```python
from build123d import *

# Parameters (mm, degrees)
BOSS_EXTRUDE1_DEPTH      = 1.5
BOSS_EXTRUDE2_DEPTH      = 18
BOSS_EXTRUDE2_DEPTH_BACK = 1
CUT_EXTRUDE2_DEPTH       = 2
CUT_EXTRUDE3_DEPTH       = 47.778734485
CHAMFER1_SIZE            = 1
CHAMFER2_SIZE            = 2


with BuildPart() as part:
    # Sketch1 → Boss-Extrude1 (new body)
    with BuildSketch(Plane(origin=(0, 0, 0), x_dir=(1, 0, 0), z_dir=(0, 1, 0))):
        Polygon((0, -2.84), (0, 0), (37, 0), (37, -6), (29, -6), (29, -10), (37, -10), (37, -16), (29, -16), (29, -28), (3, -28), (3, -2.84), align=None)
    extrude(amount=BOSS_EXTRUDE1_DEPTH)

    # Sketch2 → Boss-Extrude2 (add, two sides: drawn at the far end of the back side and taken through both)
    with BuildSketch(Plane(origin=(0, 1.5, 0), x_dir=(1, 0, 0), z_dir=(0, 1, 0)).offset(-BOSS_EXTRUDE2_DEPTH_BACK)):
        Polygon((7, 0), (0, 0), (0, -2.84), (3, -2.84), (3, -28), (7, -28), align=None)
    extrude(amount=BOSS_EXTRUDE2_DEPTH + BOSS_EXTRUDE2_DEPTH_BACK)

    # Sketch4 → Cut-Extrude2 (cut)
    with BuildSketch(Plane(origin=(7, 0, 0), x_dir=(0, 0, -1), z_dir=(1, 0, 0))):
        with BuildLine():
            Line((-17.15, 2.5), (-13.63, 2.5))
            ThreePointArc((-13.63, 2.5), (-11.508679656, 3.378679656), (-10.63, 5.5))
            Line((-10.63, 5.5), (-10.63, 15.5))
            ThreePointArc((-10.63, 15.5), (-11.508679656, 17.621320344), (-13.63, 18.5))
            Line((-13.63, 18.5), (-17.15, 18.5))
            ThreePointArc((-17.15, 18.5), (-19.271320344, 17.621320344), (-20.15, 15.5))
            Line((-20.15, 15.5), (-20.15, 5.5))
            ThreePointArc((-20.15, 5.5), (-19.271320344, 3.378679656), (-17.15, 2.5))
        make_face()
    extrude(amount=-CUT_EXTRUDE2_DEPTH, mode=Mode.SUBTRACT)

    # Sketch5 → Cut-Extrude3 (cut, through all)
    with BuildSketch(Plane(origin=(5, 0, 0), x_dir=(0, 0, -1), z_dir=(1, 0, 0))):
        with BuildLine():
            Line((-12.25, 14.75), (-12.25, 6.25))
            ThreePointArc((-12.25, 6.25), (-15.39, 3.11), (-18.53, 6.25))
            Line((-18.53, 6.25), (-18.53, 14.75))
            ThreePointArc((-18.53, 14.75), (-15.39, 17.89), (-12.25, 14.75))
        make_face()
    extrude(amount=-CUT_EXTRUDE3_DEPTH, mode=Mode.SUBTRACT)

    # Chamfer1
    chamfer1_edges = [part.edges().sort_by_distance(p)[0] for p in [
        (7, 1.5, 14),
    ]]
    chamfer(chamfer1_edges, length=CHAMFER1_SIZE - 0.0001)  # a hair under: the kernel refuses the full size

    # Chamfer2
    chamfer2_edges = [part.edges().sort_by_distance(p)[0] for p in [
        (7, 10.99995, 0),
    ]]
    chamfer(chamfer2_edges, length=CHAMFER2_SIZE)


solid = part.part
```
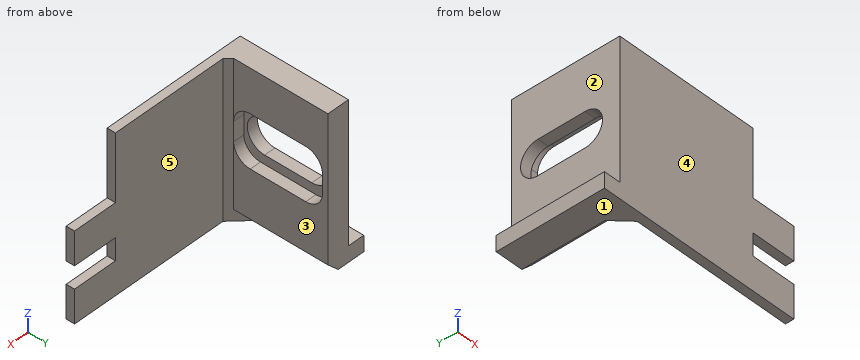
For this review, take the finished solid that the model builds, in its own axes (mm). Face numbers are marked on the shaded views. A direction names the side the tool comes from. Coordinates: 2 decimals unless noted, no trailing zeros. Write each loop counter-clockwise with the first axis right and the second up, starting at its lowest first coordinate (ties: lowest second). Pieces come first, ordered by that corner, then holes. Notation, with made-up numbers: (-5.5, 51) - (33.5, 51) arc R21 cw to (33.5, 56) - close; hole circle Ø11 at (70, 70). An arc over 180 degrees is marked (long way). Answer in a Markdown table with one row per item. Add a question column.
Q1. We need section C-C, the plane z = 9.5. State the section outline as (x, y) points.
Q2. For probe 1 along Z at (x, y) = (4, 13.25); probe 2 along Z at (x, y) = (6.5, 7.75); probe 3 along X at (y, z) = (18.5, 18), list the stretches that pass through material, from the lowest coordinate up.
Q3. Draft analysis for pull direction Y (two halves, no side actions). For the marked faces 3, 4 and 5, state which applies: +Y half, -Y half, draft (parallel to the pull), parting line (faces both ways), or undercut.
Q4. For P1, Ø8, axis at y = 9, z = 22, coming from the -X side; P2, Ø10.5, axis at y = 14.5, z = 14, coming from the +X side; P3, Ø1.2, axis at y = 1, z = 9, coming from the +X side, all flat-tipped, find the tip position at first contact; note any pin that passes through.
Q5. Tool access review of the marked faces 1 and 2: name each direction out of +Z, -Z, +X, -X, +Y, -Y from which nothing blocks a thin tool from reaching the whole face with its end or side.
Q6. We need section B-B, the plane y = 8.75. State the section outline as (x, z) points.
Q7. We need section D-D, the plane x = 21. State the section outline as (y, z) points.
Answer list:
| question | item | result |
|---|---|---|
| 1 | outline | (3, 0) - (29, 0) - (29, 1.5) - (8, 1.5) - (7, 2.5) - (7, 19.5) - (3, 19.5) - close |
| 2 | probe 1 | z = 0 to 12.25, 18.53 to 28 |
| 2 | probe 2 | z = 1.5 to 10.63, 20.15 to 28 |
| 2 | probe 3 | x = 3 to 7 |
| 3 | face 3 | draft |
| 3 | face 4 | -Y half |
| 3 | face 5 | +Y half |
| 4 | P1 | stops at x = 3 |
| 4 | P2 | stops at x = 7 |
| 4 | P3 | stops at x = 29 |
| 5 | face 1 | -Z, +X, -X, +Y, -Y |
| 5 | face 2 | +Z, -X, +Y, -Y |
| 6 | outline | (0, 0) - (5, 0) - (7, 2) - (7, 10.63) - (5, 10.63) - (5, 12.25) - (3, 12.25) - (3, 2.84) - (0, 2.84) - close; (3, 18.53) - (5, 18.53) - (5, 20.15) - (7, 20.15) - (7, 28) - (3, 28) - close |
| 7 | outline | (0, 0) - (1.5, 0) - (1.5, 28) - (0, 28) - close |
